Work out the finished part from the listing and answer in its coordinate system (mm). Give positions to 0.01 mm unless a question says otherwise; leave off trailing zeros. Write each loop counter-clockwise with the first axis right and the second up, starting at its lowest first coordinate (ties: lowest second). Pieces come first, ordered by that corner, then holes. Notation, with made-up numbers: (51, -34.5) -> (58, -34.5) arc R6 cw to (58, -30.5) -> close; hole circle Ø2 at (-8.5, 61). An arc over 180 degrees is marked (long way). Write item = value, one per line. Start each with the question number.
Solid Edge part; units mm, degrees
sketch "Sketch1" plane through (0, 0, 0) normal (0, -1, 0) x (1, 0, 0)
  line L0 (-3.1, 16.5) -> (-3.1, 23.5)
  line L1 (-32.9, 23.5) -> (-3.1, 23.5)
  line L2 (-32.9, 16.5) -> (-32.9, 23.5)
  line L3 (-32.9, 0) -> (-32.9, 16.5)
  line L4 (-32.9, 0) -> (-22.9, 0)
  line L5 (-22.9, 0) -> (-22.9, 2.5373)
  line L6 (-13.1, 2.5373) -> (-13.1, 0)
  line L7 (-13.1, 0) -> (-3.1, 0)
  line L8 (-3.1, 16.5) -> (-3.1, 0)
  arc A0 (-22.9, 2.5373) -> (-13.1, 2.5373) centre (-18, 6) cw
extrude "Protrusion1" add sketch "Sketch1" against normal blind 12
sketch "Sketch2" plane through (-18, 6, 23.5) normal (0, 0, 1) x (1, 0, 0)
  circle A0 centre (9.9, 0) radius 2.2
  circle A1 centre (-9.9, 0) radius 2.2
extrude "Cutout1" cut sketch "Sketch2" against normal through all
sketch "Sketch3" plane through (-3.1, 6, 11.75) normal (1, 0, 0) x (0, 1, 0)
  line L0 (-6, -11.75) -> (-6, 11.75)
  line L1 (6, 11.75) -> (-6, 11.75)
  line L2 (6, -11.75) -> (6, 11.75)
  line L3 (6, -11.75) -> (-6, -11.75)
extrude "ExtrudedProtrusion_2" add sketch "Sketch3" along normal blind 40
(1) Determine the mould class of faces 1 (the cylindrical face through (-25.8, 6.66, 11.91)), 2 (the flat face through (2, 0, 12)), 3 (the flat face through (36.9, 6, 12)), 4 (the cylindrical face through (-9.72, 7.49, 11.91)) for opening direction Y: pulls with the +Y half, pulls with the -Y half, needs draft (parallel to the pull), parting line crosses it, or undercut.
(2) A cutting plane is placed at D-D, the plane y = 10.5. Write down the section's boundary in (x, z).
(3) A cutting plane is placed at C-C, the plane x = -8.1. Write down the section's boundary in (y, z).
(4) Find the intervals of material crossed by line 1 along Y through (x, z) = (-28, 7.5); line 2 along X through (y, z) = (7.75, 6); line 3 along X through (y, z) = (5.25, 4.25), in increasing order.
(5) A cutting plane is placed at A-A, the plane z = 6. Write down the section's boundary in (x, y), then the cut area to 3 significant figures.
(6) A cutting plane is placed at B-B, the plane y = 6. Write down the section's boundary in (x, z), then the cut area to 3 significant figures.
Results list:
q1.face_1 = undercut
q1.face_2 = pulls with the -Y half
q1.face_3 = needs draft
q1.face_4 = undercut
q2.outline = (-32.9, 0) -> (-22.9, 0) -> (-22.9, 2.54) arc R6 cw (long way) to (-13.1, 2.54) -> (-13.1, 0) -> (36.9, 0) -> (36.9, 23.5) -> (-32.9, 23.5) -> close
q3.outline = (0, 0) -> (3.8, 0) -> (3.8, 23.5) -> (0, 23.5) -> close; (8.2, 0) -> (12, 0) -> (12, 23.5) -> (8.2, 23.5) -> close
q4.line_1 = 0 to 3.8, 8.2 to 12
q4.line_2 = -32.9 to -29.23, -26.57 to -24, -12 to -9.43, -6.77 to 36.9
q4.line_3 = -32.9 to -29.97, -25.83 to -23.74, -12.26 to -10.17, -6.03 to 36.9
q5.outline = (-32.9, 0) -> (-24, 0) -> (-24, 12) -> (-32.9, 12) -> close; (-12, 0) -> (36.9, 0) -> (36.9, 12) -> (-12, 12) -> close; hole circle Ø4.4 at (-27.9, 6); hole circle Ø4.4 at (-8.1, 6)
q5.area = 663 mm²
q6.outline = (-32.9, 0) -> (-30.1, 0) -> (-30.1, 23.5) -> (-32.9, 23.5) -> close; (-25.7, 0) -> (-22.9, 0) -> (-22.9, 2.54) arc R6 cw (long way) to (-13.1, 2.54) -> (-13.1, 0) -> (-10.3, 0) -> (-10.3, 23.5) -> (-25.7, 23.5) -> close; (-5.9, 0) -> (36.9, 0) -> (36.9, 23.5) -> (-5.9, 23.5) -> close
q6.area = 1,310 mm²
